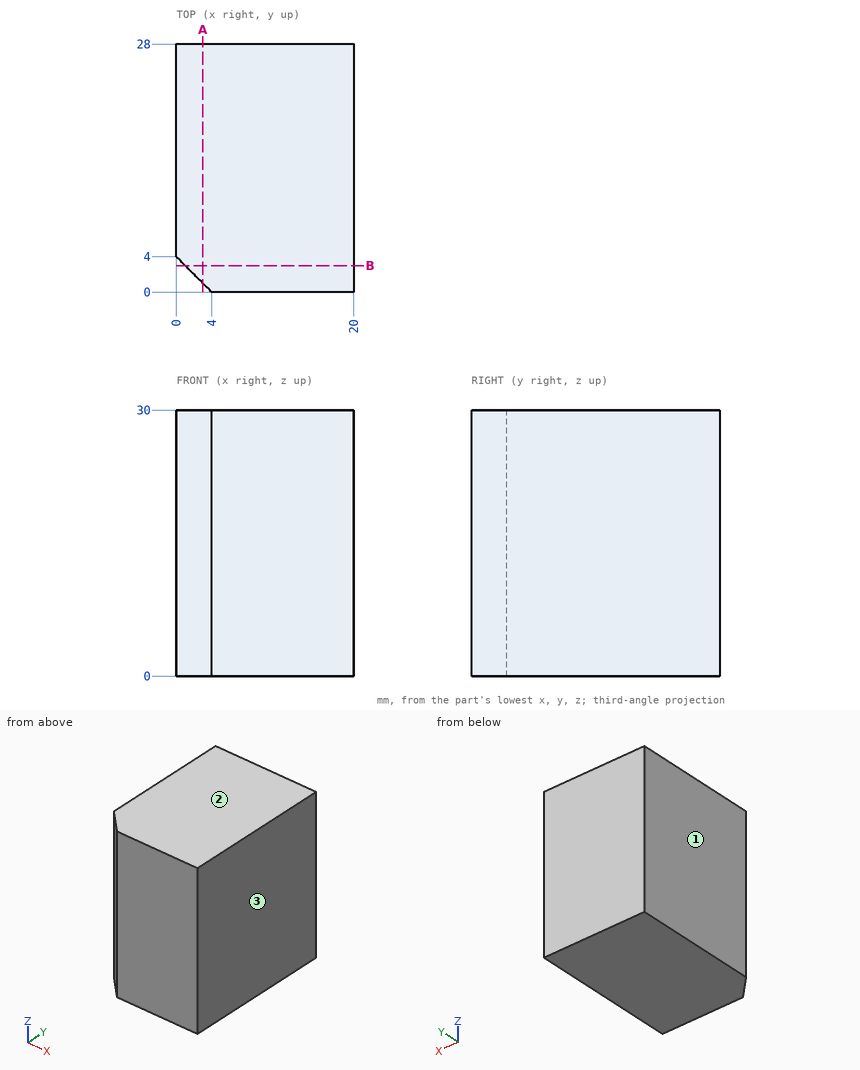
Could you check a few things on this drawing? It's one solid part, dimensions in mm from its lowest x, y, z. Round coordinates to 2 decimals unless told otherwise and drop trailing zeros. Order: outer loops, then holes, each group sorted by start corner. A loop starts at its lowest first (then second) coordinate and runs counter-clockwise, first axis right, second up. Notation, with made-up numbers: M -28,89 L -18,89 A15 cw -18,102 Z; hole C -32.5,-5 d6. An arc over 180 degrees is marked long. One line per question, with ' | ' between items. Start each with the question number.
(1) Suppose I cut it at B-B on y = 3. List the corners of the cut face in (x, z) for me.
(2) Thinking about a two-plate mould opening in X: for the marked faces 1, 2 and 3, which applies, +X half, -X half, draft (parallel to the pull), parting line (faces both ways), or undercut?
(3) For P1, Ø2, axis at x = 8.5, y = 10, coming from the -Z side, with a flat end and sliding along its axis, tell me the tip position at first contact or that it passes through.
(4) Suppose I cut it at A-A on x = 3. List the corners of the cut face in (y, z) for me, then the cut area to 3 significant figures.
(5) Please list where these lines run through material, in increasing order: line 1 along Y through (x, z) = (3.75, 6); line 2 along Y through (x, z) = (1, 28.25); line 3 along X through (y, z) = (3, 27.75).
Geometry results:
1) outline: M 1,0 L 20,0 L 20,30 L 1,30 Z
2) face 1: -X half | face 2: draft | face 3: +X half
3) P1: z = 0
4) outline: M 1,0 L 28,0 L 28,30 L 1,30 Z | area: 810 mm²
5) line 1: 0.25 to 28 | line 2: 3 to 28 | line 3: 1 to 20
